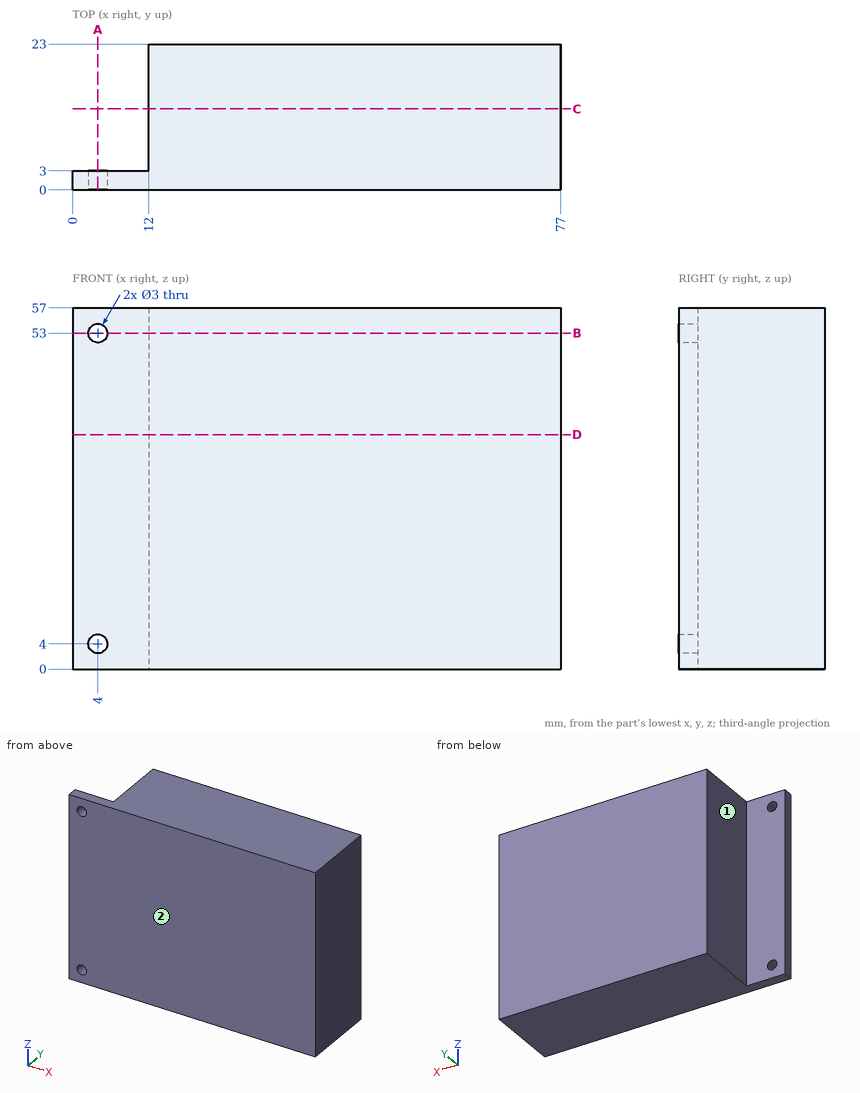
Geometry check sheet. Reference: drawing and pictorial views, mm from the part's lowest x, y, z. A direction names the side the tool comes from. Round coordinates to 2 decimals unless told otherwise and drop trailing zeros. Write each loop counter-clockwise with the first axis right and the second up, starting at its lowest first coordinate (ties: lowest second). Pieces come first, ordered by that corner, then holes. Notation, with made-up numbers: (-25, -9) -> (14, -9) arc R29 cw to (14, 26) -> close; hole circle Ø4 at (-9, 79). An arc over 180 degrees is marked (long way). Put each result on its own line as item: value.
1) Cross-section at B-B, the plane z = 53. Enter the section's corners in (x, y), plus the area to 3 significant figures.
Recorded:
outline: (0, 0) -> (2.5, 0) -> (2.5, 3) -> (0, 3) -> close; (5.5, 0) -> (77, 0) -> (77, 23) -> (12, 23) -> (12, 3) -> (5.5, 3) -> close
area: 1,520 mm2
2) Access from +Z, -Z, +X, -X, +Y, -Y to the whole of each face (thin tool, end or side, straight path). Record for the marked faces 1 and 2.
Recorded:
face 1: +Z, -Z, -X, +Y
face 2: +Z, -Z, +X, -X, -Y
3) Thickness scan on probe 1 along X at (y, z) = (1.3, 4); probe 2 along X at (y, z) = (9.5, 49). Record the ranges inside material, lowest first. Write a range as from..to.
Recorded:
probe 1: x = 0..2.5, 5.5..77
probe 2: x = 12..77
4) Depth check by flat-ended pin: P1, Ø10, axis at y = 15, z = 29.5, coming from the -X side; P2, Ø2.5, axis at x = 4, z = 4, coming from the -Y side; P3, Ø3.5, axis at x = 7.5, z = 16, coming from the +Y side. Enter the tip coordinate at first touch or a pass-through.
Recorded:
P1: stops at x = 12
P2: passes through
P3: stops at y = 3
5) Cross-section at D-D, the plane z = 37. Enter the section's corners in (x, y), plus the area to 3 significant figures.
Recorded:
outline: (0, 0) -> (77, 0) -> (77, 23) -> (12, 23) -> (12, 3) -> (0, 3) -> close
area: 1,530 mm2
6) Cross-section at C-C, the plane y = 12.75. Enter the section's corners in (x, z).
Recorded:
outline: (12, 0) -> (77, 0) -> (77, 57) -> (12, 57) -> close
7) Cross-section at A-A, the plane x = 4. Enter the section's corners in (y, z), plus the area to 3 significant figures.
Recorded:
outline: (0, 0) -> (3, 0) -> (3, 2.5) -> (0, 2.5) -> close; (0, 5.5) -> (3, 5.5) -> (3, 51.5) -> (0, 51.5) -> close; (0, 54.5) -> (3, 54.5) -> (3, 57) -> (0, 57) -> close
area: 153 mm2
